Design review of the part built by this model. Coordinates are the model's own, in mm. A direction names the side the tool comes from. Round coordinates to 2 decimals unless told otherwise and drop trailing zeros. Write each loop counter-clockwise with the first axis right and the second up, starting at its lowest first coordinate (ties: lowest second). Pieces come first, ordered by that corner, then holes. Notation, with made-up numbers: M 25,62.25 L 49,62.25 A12 cw 49,81.25 Z; hole C 83.5,-27 d10. An arc over 180 degrees is marked long. One line per question, with ' | ' between items. Start each with the question number.
Item 1: Draft analysis for pull direction Y (two halves, no side actions). For faces 1 (the face through (-18.108, -38.833, 10.876)), 2 (the face through (-18.108, 38.833, 10.876)), 3 (the face through (13.38, -25.73, 26.72)), state which applies: released by +Y, released by -Y, zero draft, split by the parting line, or undercut.
Item 2: Add section B-B, the plane x = 0. Give the number of separate pieces and of enclosed holes in the cut face, and give its area (3 significant figures).
Item 3: Machinability: for faces 4 (the face through (42.685, 3.734, 10.876)), 5 (the face through (0, -40, 16)), 6 (the face through (24.576, 35.099, 10.876)), which of the approach directions +Z, -Z, +X, -X, +Y, -Y give a long, thin tool a straight path to every point of the face, cutting with its end or side? Answer none if there is none.
Item 4: Insertion check: pin 1 Ø4 at (x, y) = (31.82, 31.82) entering from +Z; pin 2 Ø4 at (x, z) = (24.5, 24.5) entering from -Y; pin 3 Ø1.5 at (x, z) = (11.5, 14) entering from +Y; pin 4 Ø2.5 at (x, y) = (31.82, -31.82) entering from -Z. Each pin has a flat end and moves straight along its axis. Give the tip position at first contact, or say it passes through.
Item 5: For L1, parallel to Y at x = 0, z = 1.1; L2, parallel to Y at x = 0, z = 27.3; L3, parallel to Y at x = -24, z = 17, list the stretches that pass through material, from the lowest coordinate up.
Item 6: Add section C-C, the plane z = 2. State the section outline as (x, y) points, and give its area (3 significant figures).
Item 7: Add section A-A, the plane y = 0. State the section outline as (x, z) points.
```python
from build123d import *

# Parameters (mm, degrees)
SKETCH_1_R               = 40
SKETCH_1_R_2             = 35.15
EXTRUDE_1_DEPTH          = 28.2
SKETCH_2_R               = 35.5
SKETCH_2_R_2             = 29
EXTRUDE_2_DEPTH          = 5
SKETCH_3_R               = 50
SKETCH_3_R_2             = 40
EXTRUDE_3_DEPTH          = 5
SKETCH_4_R               = 1.6
CUT_EXTRUDE_1_DEPTH      = 75.419352322
FILLET_1_R               = 1.5
FILLET_2_R               = 2
REVOLVE_1_ANGLE          = 10
PATTERN_CIRCULAR_1_COUNT = 6
FILLET_3_R               = 1.5


with BuildPart() as part:
    # 草图1 → 凸台-拉伸1 (new body)
    with BuildSketch(Plane.XY):
        Circle(SKETCH_1_R)
        Circle(SKETCH_1_R_2, mode=Mode.SUBTRACT)
    extrude(amount=EXTRUDE_1_DEPTH)

    # 草图2 → 凸台-拉伸2 (add)
    with BuildSketch(Plane.XY.offset(28.2)):
        Circle(SKETCH_2_R)
        Circle(SKETCH_2_R_2, mode=Mode.SUBTRACT)
    extrude(amount=-EXTRUDE_2_DEPTH)

    # 草图3 → 凸台-拉伸3 (add)
    with BuildSketch(Plane(origin=(0, 0, 0), x_dir=(-1, 0, 0), z_dir=(0, 0, -1))):
        Circle(SKETCH_3_R)
        Circle(SKETCH_3_R_2, mode=Mode.SUBTRACT)
    extrude(amount=-EXTRUDE_3_DEPTH)

    # 草图4 → 切除-拉伸1 (cut, through all)
    with BuildSketch(Plane.XY.offset(5)):
        with Locations((31.819805153, 31.819805153)):
            Circle(SKETCH_4_R)
        with Locations((31.819805153, -31.819805153)):
            Circle(SKETCH_4_R)
        with Locations((-31.819805153, -31.819805153)):
            Circle(SKETCH_4_R)
        with Locations((-31.819805153, 31.819805153)):
            Circle(SKETCH_4_R)
        with Locations((0, 45)):
            Circle(SKETCH_4_R)
        with Locations((0, -45)):
            Circle(SKETCH_4_R)
    extrude(amount=-CUT_EXTRUDE_1_DEPTH, mode=Mode.SUBTRACT)

    # 圆角1
    fillet_1_edges = [part.edges().sort_by_distance(p)[0] for p in [
        (-35.15, 0, 23.2),
        (-40, 0, 28.2),
    ]]
    fillet(fillet_1_edges, radius=FILLET_1_R)

    # 圆角2
    fillet_2_edges = [part.edges().sort_by_distance(p)[0] for p in [
        (-29, 0, 23.2),
    ]]
    fillet(fillet_2_edges, radius=FILLET_2_R)

    # 草图5 → 旋转1 (revolve, symmetric)
    with BuildSketch(Plane(origin=(0, 0, 0), x_dir=(1, 0, 0), z_dir=(0, 1, 0))) as revolve_1_sk:
        Polygon((-50, -5), (-40, -26.7), (-40, -5), align=None)
    revolve_1 = revolve(axis=Axis((0, 0, -1.41), (0, 0, 1)), revolution_arc=REVOLVE_1_ANGLE / 2)
    revolve_1 = revolve_1 + revolve(revolve_1_sk.sketch, axis=Axis((0, 0, -1.41), (0, 0, -1)), revolution_arc=REVOLVE_1_ANGLE / 2)

    # 阵列(圆周)1: 旋转1 ×6 about axis
    pattern_circular_1_axis = Axis((0, 0, 0), (0, 0, 1))
    for i in range(1, PATTERN_CIRCULAR_1_COUNT):
        add(revolve_1.rotate(pattern_circular_1_axis, i * 360 / PATTERN_CIRCULAR_1_COUNT))

    # 圆角3
    fillet_3_edges = [part.edges().sort_by_distance(p)[0] for p in [
        (34.641016151, 20, 5),
        (0, 40, 5),
        (-34.641016151, 20, 5),
        (-34.641016151, -20, 5),
        (0, -40, 5),
        (34.641016151, -20, 5),
    ]]
    fillet(fillet_3_edges, radius=FILLET_3_R)


solid = part.part
```
Computed values:
1) face 1: released by -Y | face 2: released by +Y | face 3: undercut
2) separate pieces: 4 | enclosed holes: 0 | area: 402 mm^2
3) face 4: +Z, +Y | face 5: +Z, -Y | face 6: +Z, +X
4) pin 1: stops at z = 5 | pin 2: stops at y = -34.69 | pin 3: stops at y = 38.53 | pin 4: passes through
5) L1: y = -50 to -46.6, -43.4 to -35.15, 35.15 to 43.4, 46.6 to 50 | L2: y = -39.87 to -29, 29 to 39.87 | L3: y = -37.44 to -34.28, -32 to -25.68, 25.68 to 32, 34.28 to 37.44
6) outline: C 0,0 d100; hole C 0,0 d70.3; hole C -31.82,-31.82 d3.2; hole C -31.82,31.82 d3.2; hole C 0,-45 d3.2; hole C 0,45 d3.2; hole C 31.82,-31.82 d3.2; hole C 31.82,31.82 d3.2 | area: 3,920 mm^2
7) outline: M -50,0 L -35.15,0 L -35.15,21.7 A1.5 cw -33.65,23.2 L -31,23.2 A2 ccw -29,25.2 L -29,28.2 L -38.5,28.2 A1.5 ccw -40,26.7 L -50,5 Z; M 29,25.2 A2 ccw 31,23.2 L 33.65,23.2 A1.5 cw 35.15,21.7 L 35.15,0 L 50,0 L 50,5 L 40,26.7 A1.5 ccw 38.5,28.2 L 29,28.2 Z
